The figure shows three views and two pictorial views of one solid part (mm, origin at its lowest corner). Answer the questions. A direction names the side the tool comes from. Give positions to 0.01 mm unless a question says otherwise; leave off trailing zeros. Order: outer loops, then holes, each group sorted by start corner. A loop starts at its lowest first (then second) coordinate and runs counter-clockwise, first axis right, second up. Notation, with made-up numbers: (30.25, -38.5) - (73.25, -38.5) arc R33 ccw to (73.25, 0.5) - close; hole circle Ø10 at (13, 57.5). An arc over 180 degrees is marked (long way). Use a Markdown table: item, result. Add a question column.
1. A cutting plane is placed at B-B on x = 23. Determine the outline of the cut face in (y, z).
2. A cutting plane is placed at C-C on x = 14. Determine the outline of the cut face in (y, z), and give its area (3 significant figures).
3. Flat-ended cylindrical pins translate along their axes: P1, Ø1, axis at x = 10.5, y = 2, coming from the -Z side; P2, Ø1.2, axis at x = 2, z = 22, coming from the +Y side; P3, Ø3, axis at y = 2.5, z = 7.5, coming from the +X side. Find the tip coordinate at first contact, or state that the pin passes through.
4. Consider L1, parallel to Z at x = 2, y = 5.7; L2, parallel to Z at x = 12, y = 2.55; L3, parallel to Y at x = 15.25, z = 16.75. Determine where each line is inside the solid, lowest interval first.
5. A cutting plane is placed at D-D on z = 12.25. Determine the outline of the cut face in (x, y), and give its area (3 significant figures).
6. A cutting plane is placed at A-A on z = 22. Determine the outline of the cut face in (x, y).
7. Which of the six approach directions +Z, -Z, +X, -X, +Y, -Y give full straight-line access (tool end or side, diameter ignored) to the marked faces 1, 2 and 3?
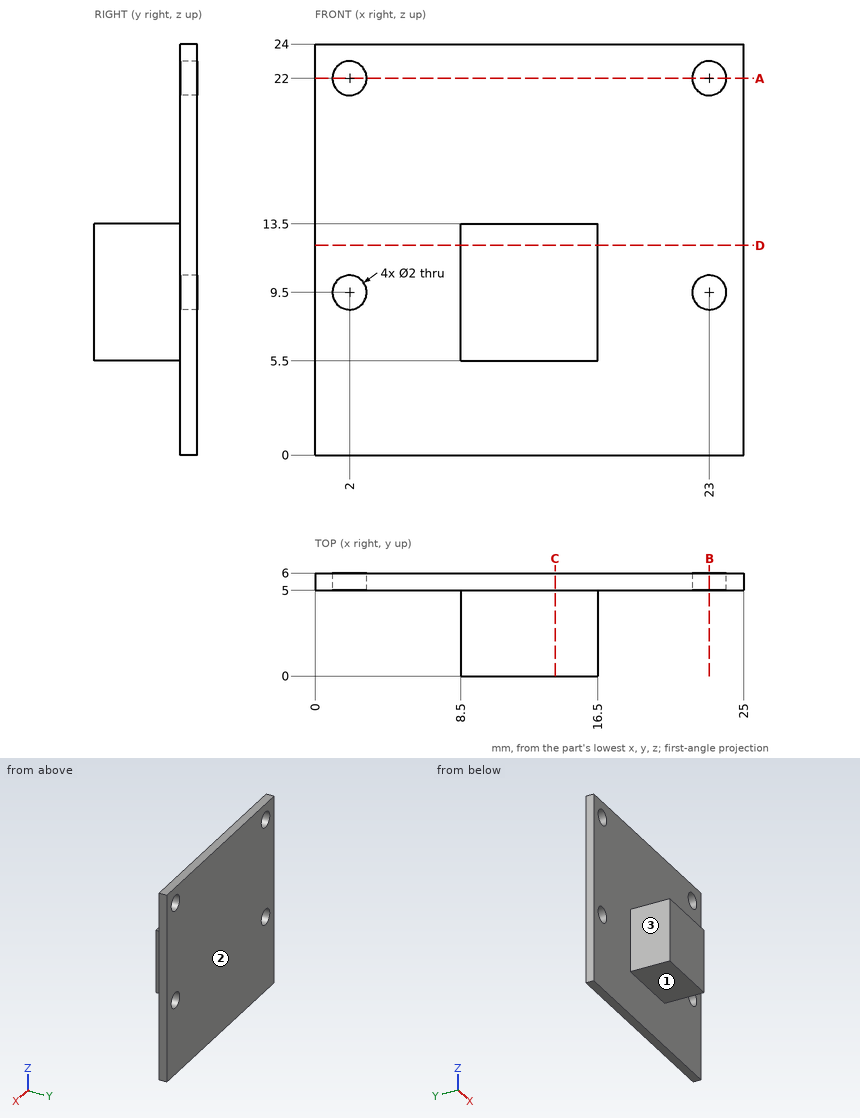
Output values:
| question | item | result |
|---|---|---|
| 1 | outline | (5, 0) - (6, 0) - (6, 8.5) - (5, 8.5) - close; (5, 10.5) - (6, 10.5) - (6, 21) - (5, 21) - close; (5, 23) - (6, 23) - (6, 24) - (5, 24) - close |
| 2 | outline | (0, 5.5) - (5, 5.5) - (5, 0) - (6, 0) - (6, 24) - (5, 24) - (5, 13.5) - (0, 13.5) - close |
| 2 | area | 64.0 mm² |
| 3 | P1 | z = 5.5 |
| 3 | P2 | through |
| 3 | P3 | x = 16.5 |
| 4 | L1 | 0 to 8.5, 10.5 to 21, 23 to 24 |
| 4 | L2 | 5.5 to 13.5 |
| 4 | L3 | 5 to 6 |
| 5 | outline | (0, 5) - (8.5, 5) - (8.5, 0) - (16.5, 0) - (16.5, 5) - (25, 5) - (25, 6) - (0, 6) - close |
| 5 | area | 65.0 mm² |
| 6 | outline | (0, 5) - (1, 5) - (1, 6) - (0, 6) - close; (3, 5) - (22, 5) - (22, 6) - (3, 6) - close; (24, 5) - (25, 5) - (25, 6) - (24, 6) - close |
| 7 | face 1 | -Z, +X, -X, -Y |
| 7 | face 2 | +Z, -Z, +X, -X, +Y |
| 7 | face 3 | +Z, -Z, -X, -Y |
